```python
from build123d import *

# Parameters (mm, degrees)
Y_KSEKLIK_EKSTR_ZYON2_DEPTH = 50
IZIM3_R                     = 45
Y_KSEKLIK_EKSTR_ZYON3_DEPTH = 210
IZIM4_R                     = 37.5
Y_KSEKLIK_EKSTR_ZYON4_DEPTH = 135
RADYUS1_R                   = 10


with BuildPart() as part:
    # Çizim1 → Döndür1 (revolve)
    with BuildSketch(Plane(origin=(0, 0, 0), x_dir=(0, 0, -1), z_dir=(1, 0, 0)), mode=Mode.PRIVATE) as d_nd_r1_sk:
        Polygon((0, 0), (0, 60), (64, 60), (64, 50), (79, 50), (79, 45), (179, 45), (179, 0), align=None)
    revolve(d_nd_r1_sk.sketch.rotate(Axis((0, 0, 55.580802483), (0, 0, -1)), 90), axis=Axis((0, 0, 55.580802483), (0, 0, -1)))

    # Çizim2 → Yükseklik-Ekstrüzyon2 (add)
    with BuildSketch(Plane.XY):
        with BuildLine():
            Line((34.344942753, 49.19781405), (312.984226436, -145.319979709))
            ThreePointArc((312.984226436, -145.319979709), (325.22389765, -206.324838294), (264.818131867, -221.242806741))
            Line((264.818131867, -221.242806741), (-29.876516673, -52.032621993))
            Line((-29.876516673, -52.032621993), (34.344942753, 49.19781405))
        make_face()
    extrude(amount=-Y_KSEKLIK_EKSTR_ZYON2_DEPTH)

    # Çizim3 → Yükseklik-Ekstrüzyon3 (add)
    with BuildSketch(Plane(origin=(0, 0, -50), x_dir=(-1, 0, 0), z_dir=(0, 0, -1))):
        with Locations(Location((-287.225519371, -182.218340246, 0), (0, 0, 124.918853114))):
            Circle(IZIM3_R)
    extrude(amount=-Y_KSEKLIK_EKSTR_ZYON3_DEPTH)

    # Çizim4 → Yükseklik-Ekstrüzyon4 (add)
    with BuildSketch(Plane.XY.offset(160)):
        with Locations((287.225519371, -182.218340246)):
            Circle(IZIM4_R)
    extrude(amount=Y_KSEKLIK_EKSTR_ZYON4_DEPTH)

    # Radyus1
    radyus1_edges = [part.edges().sort_by_distance(p)[0] for p in [
        (249.725519371, -182.218340246, 295),
        (-45, 0, -179),
    ]]
    fillet(radyus1_edges, radius=RADYUS1_R)


solid = part.part
```
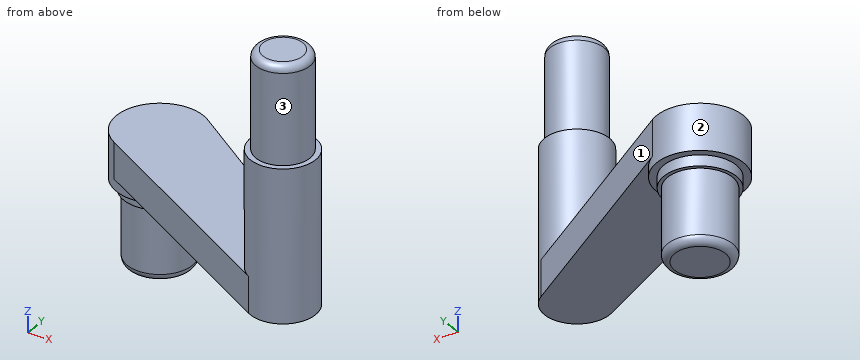
Geometry check sheet. Reference: the model listing, model coordinates, mm. Face numbers are marked on the shaded views. A direction names the side the tool comes from. Give positions to 0.01 mm unless a question says otherwise; leave off trailing zeros. Loops run counter-clockwise (first coordinate to the right, second up) from the corner with the lowest first, then second, coordinate; pieces in that order, holes last. Notation, with made-up numbers: M -17,-28 L -4,-28 A21 ccw -4,-13 Z; hole C 43.5,-5.5 d10. An arc over 180 degrees is marked long. Write item = value, one per line. Start each with the question number.
1. Section check D-D, the plane z = 24.5. Enter the section's corners in (x, y).
2. Section check A-A, the plane x = 0. Enter the section's corners in (y, z).
3. Thickness scan on probe 1 along Z at (x, y) = (153.5, -48); probe 2 along Z at (x, y) = (-29, 9); probe 3 along X at (y, z) = (27, -2.5). Record the ranges inside material, lowest first.
4. Section check B-B, the plane y = 0. Enter the section's corners in (x, z).
5. Go/stop test with flat-tipped pins: P1, Ø1, axis at y = -166.5, z = -10, coming from the +X side; P2, Ø1.5, axis at x = 185.5, y = -107, coming from the +Z side. Record where each tip stops, or that it passes through.
6. Tool access check on the marked faces 1, 2 and 3. Record the directions out of +Z, -Z, +X, -X, +Y, -Y that give a thin tool (end or side, any length) a straight path to the whole face; none if there is none.
7. Section check C-C, the plane z = 221.5. Enter the section's corners in (x, y).
Values follow:
q1.outline = C 287.23,-182.22 d90
q2.outline = M -69.19,-50 L -60,-50 L -60,-64 L -50,-64 L -50,-79 L -45,-79 L -45,-169 A10 ccw -35,-179 L 35,-179 A10 ccw 45,-169 L 45,-79 L 50,-79 L 50,-64 L 60,-64 L 60,0 L -69.19,0 Z
q3.probe_1 = -50 to 0
q3.probe_2 = -179 to 0
q3.probe_3 = -53.58 to 66.14
q4.outline = M -60,-64 L -50,-64 L -50,-79 L -45,-79 L -45,-169 A10 ccw -35,-179 L 35,-179 A10 ccw 45,-169 L 45,-79 L 50,-79 L 50,-64 L 60,-64 L 60,-50 L 104.82,-50 L 104.82,0 L -60,0 Z
q5.P1 = 329.57
q5.P2 = 0
q6.face_1 = +Z, -Z, +X, +Y
q6.face_2 = -Z
q6.face_3 = +Z
q7.outline = C 287.23,-182.22 d75
